from build123d import *

# Parameters (mm, degrees)
SALIENTE_EXTRUIR2_DEPTH = 228.6
REDONDEO1_R             = 2
CROQUIS3_R              = 5
CORTAR_EXTRUIR1_DEPTH   = 151
SALIENTE_EXTRUIR3_START = -3
CROQUIS5_W              = 50
CROQUIS5_H              = 2
SALIENTE_EXTRUIR3_DEPTH = 53
CROQUIS6_R              = 5
CORTAR_EXTRUIR2_DEPTH   = 50
SALIENTE_EXTRUIR4_DEPTH = 2
CROQUIS8_W              = 5
CROQUIS8_H              = 10
CORTAR_EXTRUIR3_DEPTH   = 10


with BuildPart() as part:
    # Croquis2 → Saliente-Extruir2 (new body, symmetric)
    with BuildSketch(Plane.XY):
        Polygon((-75, 20), (-55, 20), (-55, 18), (-73, 18), (-73, -18), (73, -18), (73, 18), (55, 18), (55, 20), (75, 20), (75, -20), (-75, -20), align=None)
    extrude(amount=SALIENTE_EXTRUIR2_DEPTH, both=True)

    # Redondeo1
    redondeo1_edges = [part.edges().sort_by_distance(p)[0] for p in [
        (75, 20, 0),
        (75, -20, 0),
        (-75, -20, 0),
        (-75, 20, 0),
        (-73, 18, 0),
        (-73, -18, 0),
        (73, -18, 0),
        (73, 18, 0),
    ]]
    fillet(redondeo1_edges, radius=REDONDEO1_R)

    # Croquis3 → Cortar-Extruir1 (cut, through all)
    with BuildSketch(Plane(origin=(75, 0, 0), x_dir=(0, 0, -1), z_dir=(1, 0, 0))):
        with Locations((-211.1, 0)):
            Circle(CROQUIS3_R)
    extrude(amount=-CORTAR_EXTRUIR1_DEPTH, mode=Mode.SUBTRACT)

    # Croquis5 → Saliente-Extruir3 (add)
    with BuildSketch(Plane(origin=(75, 0, 0), x_dir=(0, 0, -1), z_dir=(1, 0, 0)).offset(SALIENTE_EXTRUIR3_START)):
        with Locations((-53.6, -19)):
            Rectangle(CROQUIS5_W, CROQUIS5_H)
    saliente_extruir3 = extrude(amount=SALIENTE_EXTRUIR3_DEPTH)

    # Croquis6 → Cortar-Extruir2 (cut)
    with BuildSketch(Plane(origin=(0, -18, 0), x_dir=(1, 0, 0), z_dir=(0, 1, 0))):
        with Locations((105, -53.6)):
            Circle(CROQUIS6_R)
    cortar_extruir2 = extrude(amount=-CORTAR_EXTRUIR2_DEPTH, mode=Mode.SUBTRACT)

    # Croquis7 → Saliente-Extruir4 (add)
    with BuildSketch(Plane(origin=(0, 0, 28.6), x_dir=(-1, 0, 0), z_dir=(0, 0, -1))):
        Polygon((-75, -18), (-75, 18), (-125, -18), align=None)
    saliente_extruir4 = extrude(amount=-SALIENTE_EXTRUIR4_DEPTH)

    # Simetría1: Saliente-Extruir3, Cortar-Extruir2, Saliente-Extruir4 across plane
    add(saliente_extruir3.mirror(Plane(origin=(0, 0, 0), x_dir=(0, 0, 1), z_dir=(1, 0, 0))))
    add(cortar_extruir2.mirror(Plane(origin=(0, 0, 0), x_dir=(0, 0, 1), z_dir=(1, 0, 0))), mode=Mode.SUBTRACT)
    add(saliente_extruir4.mirror(Plane(origin=(0, 0, 0), x_dir=(0, 0, 1), z_dir=(1, 0, 0))))

    # Croquis8 → Cortar-Extruir3 (cut)
    with BuildSketch(Plane(origin=(0, 20, 0), x_dir=(1, 0, 0), z_dir=(0, 1, 0))):
        with Locations((-57.5, 0.1)):
            Rectangle(CROQUIS8_W, CROQUIS8_H)
        with Locations((57.5, 0.1)):
            Rectangle(CROQUIS8_W, CROQUIS8_H)
    extrude(amount=-CORTAR_EXTRUIR3_DEPTH, mode=Mode.SUBTRACT)


solid = part.part
Check sheet for the modelled part. Datum: model origin and axes. Units: mm. A direction names the side the tool comes from. Give positions to 0.01 mm unless a question says otherwise; leave off trailing zeros. Loops run counter-clockwise (first coordinate to the right, second up) from the corner with the lowest first, then second, coordinate; pieces in that order, holes last. Notation, with made-up numbers: M 74.25,19.5 L 132.25,19.5 A4 cw 132.25,25.5 Z; hole C 7,-37 d10. An arc over 180 degrees is marked long. Use a Markdown table: item, result. Add a question column.
Q1. Scan lines: line 1 along X through (y, z) = (-19.6, 53.6); line 2 along X through (y, z) = (-9.5, -46); line 3 along X through (y, z) = (16.5, 79.5). Record each from-to range of solid material in increasing order. Write a range as [from, to].
Q2. Sectioned sample at A-A, the plane x = 105. Record the cut outline in (y, z), then the cut area to 3 significant figures.
Q3. Sectioned sample at B-B, the plane y = 0. Record the cut outline in (x, z), then the cut area to 3 significant figures.
Q4. Mould release check, pull along Y, two halves, no side actions. Record for faces 1 (the flat face through (2, -20, 3)), 2 (the cylindrical face through (74.01, 1.5, 206.33)), 3 (the flat face through (100, -18, 55)): pulls with the +Y half, pulls with the -Y half, needs draft (parallel to the pull), parting line crosses it, or undercut.
Q5. Sectioned sample at C-C, the plane z = 211.1. Record the cut outline in (x, y), then the cut area to 3 significant figures.
Q6. Tool access check on faces 4 (the flat face through (-89, -8, 30.6)), 5 (the flat face through (75, 0, 131)), 6 (the cylindrical face through (-73.99, 1.5, 206.33)), 7 (the flat face through (73, 0, 3)). Record the directions out of +Z, -Z, +X, -X, +Y, -Y that give a thin tool (end or side, any length) a straight path to the whole face; none if there is none.
Q7. Sectioned sample at D-D, the plane z = 53.6. Give the number of separate pieces and of enclosed holes in the cut face, then the cut area to 3 significant figures.
Q8. Go/stop test with flat-tipped pins: pin 1 (10 mm diameter, centred on x = 81, z = 117.5, fed in from +Y); pin 2 (2 mm diameter, centred on x = -93.5, y = -19, fed in from +Z); pin 3 (1 mm diameter, centred on y = 19, z = -69.5, fed in from +X); pin 4 (2 mm diameter, centred on y = 19, z = 132.5, fed in from +X). Record where each tip stops, or that it passes through.
Verdict:
| question | item | result |
|---|---|---|
| 1 | line 1 | [-125, -110], [-100, 100], [110, 125] |
| 1 | line 2 | [-75, -73], [73, 75] |
| 1 | line 3 | [-75, -72.94], [72.94, 75] |
| 2 | outline | M -20,28.6 L -3.6,28.6 L -3.6,30.6 L -18,30.6 L -18,48.6 L -20,48.6 Z; M -20,58.6 L -18,58.6 L -18,78.6 L -20,78.6 Z |
| 2 | area | 109 mm^2 |
| 3 | outline | M -100,28.6 L -75,28.6 L -75,-228.6 L -73,-228.6 L -73,206.1 L -75,206.1 L -75,30.6 L -100,30.6 Z; M -75,216.1 L -73,216.1 L -73,228.6 L -75,228.6 Z; M 73,-228.6 L 75,-228.6 L 75,28.6 L 100,28.6 L 100,30.6 L 75,30.6 L 75,206.1 L 73,206.1 Z; M 73,216.1 L 75,216.1 L 75,228.6 L 73,228.6 Z |
| 3 | area | 1,890 mm^2 |
| 4 | face 1 | pulls with the -Y half |
| 4 | face 2 | undercut |
| 4 | face 3 | pulls with the +Y half |
| 5 | outline | M -75,-18 A2 ccw -73,-20 L 73,-20 A2 ccw 75,-18 L 75,-5 L 73,-5 L 73,-16 A2 cw 71,-18 L -71,-18 A2 cw -73,-16 L -73,-5 L -75,-5 Z; M -75,5 L -73,5 L -73,16 A2 cw -71,18 L -55,18 L -55,20 L -73,20 A2 ccw -75,18 Z; M 55,18 L 71,18 A2 cw 73,16 L 73,5 L 75,5 L 75,18 A2 ccw 73,20 L 55,20 Z |
| 5 | area | 484 mm^2 |
| 6 | face 4 | +Z, -X, +Y |
| 6 | face 5 | +Z, +X, +Y |
| 6 | face 6 | +X, -X |
| 6 | face 7 | +Z, -Z |
| 7 | separate pieces | 3 |
| 7 | enclosed holes | 0 |
| 7 | area | 686 mm^2 |
| 8 | pin 1 | through |
| 8 | pin 2 | z = 78.6 |
| 8 | pin 3 | x = 74.94 |
| 8 | pin 4 | x = 75 |
